Here's how the part is built. I have some questions about the finished solid (model axes, mm). A direction names the side the tool comes from. Coordinates: 2 decimals unless noted, no trailing zeros. Answer in a Markdown table with one row per item. Add a question column.
Item 1: Which directions (+Z, -Z, +X, -X, +Y, -Y) give clear straight access to the entire face, cutting with the end or side of a thin tool? Please do faces 1 (the face through (-2.19, 8.32, 9.84)), 2 (the face through (3.721, 0.038, -9.454)).
Item 2: I'm going to push flat-ended pins straight in: pin 1 (2 mm diameter, centred on y = -3, z = -3.5, fed in from +X); pin 2 (12 mm diameter, centred on y = 8.5, z = -14, fed in from -X); pin 3 (3 mm diameter, centred on y = 0, z = 4, fed in from -X). Where does each tip first touch, or does it pass through?
Item 3: If I drill on probe 1 along X at (y, z) = (-0.25, -12); probe 2 along Y at (x, z) = (-1.25, 0); probe 3 along Z at (x, y) = (1.5, 5), over which ranges is the centre line in solid material (lowest first)? Write a range as from..to.
Item 4: Imagine slicing it at A-A (z = -9). State how many separate pieces and enclosed holes the cut face has, plus the area to 3 significant figures.
Item 5: We'd pull the mould along X, two halves only. Please class faces 3 (the face through (-8.12, 2.91, -18.64)), 4 (the face through (7.39, 2.84, -11.7)), 5 (the face through (-2.187, -11.134, -6.488)): +X half, -X half, draft (parallel to the pull), parting line (faces both ways), or undercut.
from build123d import *

# Parameters (mm, degrees)
SKETCH1_R           = 5.08
BOSS_EXTRUDE1_DEPTH = 12.7
SKETCH5_R           = 3.81
BOSS_EXTRUDE2_DEPTH = 20.32
SKETCH6_R           = 2.7305
CUT_EXTRUDE1_DEPTH  = 10.16
CUT_EXTRUDE2_REACH  = 34.362
SKETCH7_R           = 2.7305


with BuildPart() as part:
    # Sketch1 → Boss-Extrude1 (new, symmetric)
    with BuildSketch(Plane(origin=(0, 0, 0), x_dir=(1, 0, 0), z_dir=(0, 0.7660444431189771, 0.6427876096865406))):
        with Locations(Location((0, 0, 0), (0, 0, 270))):
            Circle(SKETCH1_R)
    extrude(amount=BOSS_EXTRUDE1_DEPTH, both=True)

    # Sketch5 → Boss-Extrude2 (add)
    with BuildSketch(Plane(origin=(0, 0, 0), x_dir=(0, -1, 0), z_dir=(-0.36974675727382683, 0, -0.9291325715340572))):
        with Locations(Location((0, 0, 0), (0, 0, 200.690266715))):
            Circle(SKETCH5_R)
    boss_extrude2 = extrude(amount=BOSS_EXTRUDE2_DEPTH)

    # Sketch6 → Cut-Extrude1 (cut)
    with BuildSketch(Plane(origin=(-7.513254108, 0, -18.879973854), x_dir=(-0.9291325715340572, 0, 0.36974675727382694), z_dir=(-0.3697467572738269, 0, -0.929132571534057))):
        Circle(SKETCH6_R)
    cut_extrude1 = extrude(amount=-CUT_EXTRUDE1_DEPTH, mode=Mode.SUBTRACT)

    # Mirror1: Boss-Extrude2, Cut-Extrude1 across plane
    add(boss_extrude2.mirror(Plane(origin=(0, 0, 0), x_dir=(0, 0, 1), z_dir=(1, 0, 0))))
    add(cut_extrude1.mirror(Plane(origin=(0, 0, 0), x_dir=(0, 0, 1), z_dir=(1, 0, 0))), mode=Mode.SUBTRACT)

    # Sketch7 → Cut-Extrude2 (cut, up to next)
    with BuildSketch(Plane(origin=(0, -9.728764428, -8.163402643), x_dir=(1, 0, 0), z_dir=(0, -0.7660444431189772, -0.6427876096865405)), mode=Mode.PRIVATE) as cut_extrude2_sk1:
        with Locations(Location((0, 0, 0), (0, 0, 270))):
            Circle(SKETCH7_R)
    cut_extrude2_tool1 = extrude(cut_extrude2_sk1.sketch, amount=-CUT_EXTRUDE2_REACH, mode=Mode.PRIVATE) & part.part
    add(cut_extrude2_tool1.solids().sort_by_distance((0, -9.728764, -8.163403))[0], mode=Mode.SUBTRACT)


solid = part.part
Here are the results:
| question | item | result |
|---|---|---|
| 1 | face 1 | +Z, +X, -X, +Y |
| 1 | face 2 | none |
| 2 | pin 1 | stops at x = 5.08 |
| 2 | pin 2 | stops at x = -9.1 |
| 2 | pin 3 | stops at x = -4.83 |
| 3 | probe 1 | x = -8.87..-7.7, -1.85..-0.68, 0.68..1.85, 7.7..8.87 |
| 3 | probe 2 | y = -7.66..-3.78, 3.78..7.66 |
| 3 | probe 3 | z = -2.14..1.22, 7.17..10.53 |
| 4 | separate pieces | 1 |
| 4 | enclosed holes | 3 |
| 4 | area | 120 mm2 |
| 5 | face 3 | -X half |
| 5 | face 4 | undercut |
| 5 | face 5 | draft |
